Verification items for the finished model (mm, model axes). A direction names the side the tool comes from. Give positions to 0.01 mm unless a question says otherwise; leave off trailing zeros. Loops run counter-clockwise (first coordinate to the right, second up) from the corner with the lowest first, then second, coordinate; pieces in that order, holes last. Notation, with made-up numbers: M 86.5,54.25 L 94.5,54.25 A7 cw 94.5,65.25 Z; hole C 44.5,51.25 d7. An arc over 180 degrees is marked long. Answer in a Markdown table with one row per item.
```python
from build123d import *

# Parameters (mm, degrees)
F0_W     = 18.864762
F0_H     = 50
F3_DEPTH = 100


with BuildPart() as f1:
    # F0 (on Top) → F1 (revolve)
    with BuildSketch(Plane.XY):
        with Locations((-24.432381, 75)):
            Rectangle(F0_W, F0_H)
    revolve(axis=Axis((0, 34.19238, 0), (0, -1, 0)))

    # F2 (on Front) → F3 (join)
    with BuildSketch(Plane.XZ):
        with BuildLine():
            Line((111.403681, 5), (33.493613, 5))
            ThreePointArc((33.493613, 5), (33.864762, 0), (33.493613, -5))
            Line((33.493613, -5), (111.403681, -5))
            Line((111.403681, -5), (111.403681, 5))
        make_face()
    extrude(amount=-F3_DEPTH)


solid = f1.part
```
Item 1: Sectioned sample at B-B (y = 70). Record the cut outline in (x, z), and give its area (3 significant figures).
Reported:
| item | result |
|---|---|
| outline | M 33.49,-5 L 111.4,-5 L 111.4,5 L 33.49,5 A33.86 ccw long Z; hole C 0,0 d30 |
| area | 3,670 mm^2 |
Item 2: Release check for a two-part mould opening along Z. For faces 3 (the flat face through (73, 49, 5)), 4 (the cylindrical face through (14.985, 75.35, -0.66)), 5 (the cylindrical face through (33.865, 24.65, 0.07)), 6 (the flat face through (111.404, 49, 0)) record: released by +Z, released by -Z, zero draft, split by the parting line, or undercut.
Reported:
| item | result |
|---|---|
| face 3 | released by +Z |
| face 4 | undercut |
| face 5 | undercut |
| face 6 | zero draft |
Item 3: Sectioned sample at C-C (y = 44). Record the cut outline in (x, z).
Reported:
| item | result |
|---|---|
| outline | M 33.49,-5 L 111.4,-5 L 111.4,5 L 33.49,5 A33.86 cw Z |
Item 4: Sectioned sample at A-A (x = 2). Record the cut outline in (y, z), and give its area (3 significant figures).
Reported:
| item | result |
|---|---|
| outline | M 50,-33.81 L 100,-33.81 L 100,-14.87 L 50,-14.87 Z; M 50,14.87 L 100,14.87 L 100,33.81 L 50,33.81 Z |
| area | 1,890 mm^2 |
Item 5: Go/stop test with flat-tipped pins: pin 1 (5 mm diameter, centred on x = 96.5, y = 66.5, fed in from -Z); pin 2 (1 mm diameter, centred on x = 46, y = 21.5, fed in from +Z); pin 3 (1.5 mm diameter, centred on x = 26, y = 69, fed in from +Z); pin 4 (8 mm diameter, centred on x = -11.5, z = 8, fed in from +Y). Record where each tip stops, or that it passes through.
Reported:
| item | result |
|---|---|
| pin 1 | stops at z = -5 |
| pin 2 | stops at z = 5 |
| pin 3 | stops at z = 22.57 |
| pin 4 | stops at y = 100 |
Item 6: Tool access check on faces 1 (the flat face through (17, 100, 3)), 2 (the flat face through (72, 49, -5)). Record the directions out of +Z, -Z, +X, -X, +Y, -Y that give a thin tool (end or side, any length) a straight path to the whole face; none if there is none.
Reported:
| item | result |
|---|---|
| face 1 | +Z, -Z, +X, -X, +Y |
| face 2 | -Z, +X, +Y, -Y |
Item 7: Sectioned sample at D-D (z = -17). Record the cut outline in (x, y).
Reported:
| item | result |
|---|---|
| outline | M -29.29,50 L 29.29,50 L 29.29,100 L -29.29,100 Z |
Item 8: Scan lines: L1, parallel to X at y = 66, z = 0; L2, parallel to Z at x = 0, y = 62.5; L3, parallel to Z at x = 94, y = 94.5. Record each from-to range of solid material in increasing order. Write a range as [from, to].
Reported:
| item | result |
|---|---|
| L1 | x = [-33.86, -15], [15, 111.4] |
| L2 | z = [-33.86, -15], [15, 33.86] |
| L3 | z = [-5, 5] |
